Input: part model. Units: mm. Frame: model coordinates. Face numbers are marked on the shaded views. A direction names the side the tool comes from. Round coordinates to 2 decimals unless told otherwise and drop trailing zeros. Order: outer loops, then holes, each group sorted by start corner. A loop starts at its lowest first (then second) coordinate and runs counter-clockwise, first axis right, second up. Notation, with made-up numbers: (63.5, -14) -> (92.5, -14) arc R29 ccw to (92.5, 22) -> close; hole circle Ø10 at (50.5, 36.25). An arc over 180 degrees is marked (long way). Answer as CSV lines item,"result". Start each with the question number.
1) Line query: L1, parallel to Y at x = 0, z = 3.25; L2, parallel to X at y = -1.25, z = 6.25; L3, parallel to Y at x = 7, z = 3.75. Output: solid intervals per line, ascending.
2) Section query B-B, the plane z = 4.5. Output: boundary loops of the cut face in (x, y).
3) Mould query, pull axis Y, two halves, no side actions, for the marked faces 1, 2, 3 and 4. Classes: +Y half, -Y half, draft (parallel to the pull), parting line (faces both ways), or undercut.
4) Section query A-A, the plane z = 7.5. State how many separate pieces and enclosed holes the cut face has, and give its area (3 significant figures).
5) First-contact query: P1, Ø2, axis at x = 8, y = -0.5, coming from the +Z side; P2, Ø1, axis at y = 5.5, z = 6, coming from the +X side; P3, Ø1, axis at y = 3.5, z = 4, coming from the +X side. Flat tips, straight axial feed; report the tip coordinate or a pass-through.
6) Access query for the marked faces 5, 6 and 7. Directions: +Z, -Z, +X, -X, +Y, -Y. A direction counts if a zero-diameter tool reaches every point of the face in a straight line with its end or side. Return the directions, or none.
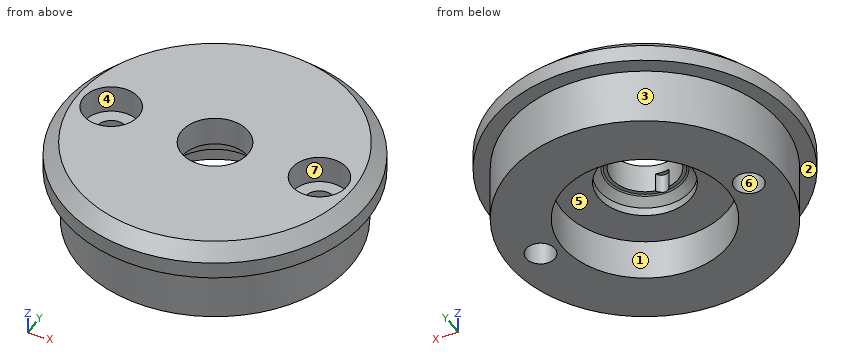
```python
from build123d import *

# Parameters (mm, degrees)
SKETCH1_R               = 9.9
BOSS_EXTRUDE1_DEPTH     = 4.1024
SKETCH3_R               = 11
BOSS_EXTRUDE2_DEPTH     = 2.2114
CUT_EXTRUDE1_DEPTH      = 17.088184663
CUT_EXTRUDE1_DEPTH_BACK = 1.5
SKETCH6_R               = 0.5
CHAMFER1_SIZE           = 1
SKETCH7_R               = 2
CUT_EXTRUDE2_DEPTH      = 2
SKETCH8_R               = 1.05
CUT_EXTRUDE3_DEPTH      = 17.143384727
SKETCH9_R               = 6.003028119
CUT_EXTRUDE4_DEPTH      = 3


with BuildPart() as part:
    # Sketch1 → Boss-Extrude1 (new body)
    with BuildSketch(Plane.XY.offset(2.5)):
        with Locations(Location((0, 0, 0), (0, 0, 180))):
            Circle(SKETCH1_R)
    extrude(amount=BOSS_EXTRUDE1_DEPTH)

    # Sketch3 → Boss-Extrude2 (add)
    with BuildSketch(Plane.XY.offset(6.6024)):
        Circle(SKETCH3_R)
    extrude(amount=BOSS_EXTRUDE2_DEPTH)

    # Sketch4 → Cut-Revolve2 (revolve, cut)
    with BuildSketch(Plane(origin=(0, 0, 0), x_dir=(0, 0, -1), z_dir=(1, 0, 0)), mode=Mode.PRIVATE) as cut_revolve2_sk:
        with BuildLine():
            Line((-6.113239385, 3.350496042), (0, 3.350496042))
            Line((0, 3.350496042), (0, 0))
            Line((0, 0), (-8.8138, 0))
            Line((-8.8138, 0), (-8.8138, 2.4225))
            Line((-8.8138, 2.4225), (-6.7024, 2.4225))
            Line((-6.7024, 2.4225), (-6.7024, 2.673729766))
            Line((-6.7024, 2.673729766), (-6.644568783, 2.814399725))
            ThreePointArc((-6.644568783, 2.814399725), (-6.379015778, 3.082558584), (-6.113239385, 3.350496042))
        make_face()
    revolve(cut_revolve2_sk.sketch.rotate(Axis((0, 0, 8.8138), (0, 0, -1)), 90), axis=Axis((0, 0, 8.8138), (0, 0, -1)), mode=Mode.SUBTRACT)

    # Sketch6 → Cut-Extrude1 (cut, two sides: drawn at the far end of the back side and taken through both)
    with BuildSketch(Plane(origin=(0, 0, 6.6024), x_dir=(-1, 0, 0), z_dir=(0, 0, -1)).offset(-CUT_EXTRUDE1_DEPTH_BACK)):
        with Locations((1.2e-08, -2.2225)):
            Circle(SKETCH6_R)
    extrude(amount=CUT_EXTRUDE1_DEPTH + CUT_EXTRUDE1_DEPTH_BACK, mode=Mode.SUBTRACT)

    # Chamfer1
    chamfer1_edges = [part.edges().sort_by_distance(p)[0] for p in [
        (-11, 0, 8.8138),
    ]]
    chamfer(chamfer1_edges, length=CHAMFER1_SIZE)

    # Sketch7 → Cut-Extrude2 (cut)
    with BuildSketch(Plane.XY.offset(8.8138)):
        with Locations((-7.549511775, 0.085860102)):
            Circle(SKETCH7_R)
        with Locations((7.55, 0)):
            Circle(SKETCH7_R)
    extrude(amount=-CUT_EXTRUDE2_DEPTH, mode=Mode.SUBTRACT)

    # Sketch8 → Cut-Extrude3 (cut, through all)
    with BuildSketch(Plane.XY.offset(6.8138)):
        with Locations((-7.549511775, 0.085860102)):
            Circle(SKETCH8_R)
        with Locations((7.55, 0)):
            Circle(SKETCH8_R)
    extrude(amount=-CUT_EXTRUDE3_DEPTH, mode=Mode.SUBTRACT)

    # Sketch9 → Cut-Extrude4 (cut)
    with BuildSketch(Plane(origin=(0, 0, 2.5), x_dir=(-1, 0, 0), z_dir=(0, 0, -1))):
        Circle(SKETCH9_R)
    extrude(amount=-CUT_EXTRUDE4_DEPTH, mode=Mode.SUBTRACT)


solid = part.part
```
Findings:
1,L1,"y = -9.9 to -6, 6 to 9.9"
1,L2,"x = -9.82 to -2.96, 2.96 to 9.82"
1,L3,"y = -7 to -0.89, 0.89 to 7"
2,outline,"circle Ø19.8 at (0, 0); hole circle Ø2.1 at (-7.55, 0.09); hole circle Ø12.01 at (0, 0); hole circle Ø2.1 at (7.55, 0)"
3,face 1,"undercut"
3,face 2,"draft"
3,face 3,"parting line"
3,face 4,"undercut"
4,separate pieces,"1"
4,enclosed holes,"3"
4,area,"336 mm^2"
5,P1,"stops at z = 6.81"
5,P2,"stops at x = 8.54"
5,P3,"stops at x = 9.43"
6,face 5,"-Z"
6,face 6,"+Z, -Z"
6,face 7,"+Z"
